```python
from build123d import *

# Parameters (mm, degrees)
SKETCH1_W           = 54
SKETCH1_H           = 32
SKETCH1_W_2         = 25
SKETCH1_H_2         = 14
BOSS_EXTRUDE1_DEPTH = 7
SKETCH2_W           = 54
SKETCH2_H           = 32
BOSS_EXTRUDE2_DEPTH = 1
CHAMFER1_SIZE       = 1


with BuildPart() as part:
    # Sketch1 → Boss-Extrude1 (new body)
    with BuildSketch(Plane(origin=(0, 0, 0), x_dir=(1, 0, 0), z_dir=(0, 1, 0))):
        with Locations((1.304347826, -0.359533527)):
            Rectangle(SKETCH1_W, SKETCH1_H)
        with Locations((-11.695652174, 7.140466473)):
            Rectangle(SKETCH1_W_2, SKETCH1_H_2, mode=Mode.SUBTRACT)
        with Locations((-11.695652174, -7.859533527)):
            Rectangle(SKETCH1_W_2, SKETCH1_H_2, mode=Mode.SUBTRACT)
        with Locations((14.304347826, 7.140466473)):
            Rectangle(SKETCH1_W_2, SKETCH1_H_2, mode=Mode.SUBTRACT)
        with Locations((14.304347826, -7.859533527)):
            Rectangle(SKETCH1_W_2, SKETCH1_H_2, mode=Mode.SUBTRACT)
    extrude(amount=BOSS_EXTRUDE1_DEPTH)

    # Sketch2 → Boss-Extrude2 (add)
    with BuildSketch(Plane.XZ):
        with Locations((1.304347826, 0.359533527)):
            Rectangle(SKETCH2_W, SKETCH2_H)
    extrude(amount=BOSS_EXTRUDE2_DEPTH)

    # Chamfer1
    chamfer1_edges = [part.edges().sort_by_distance(p)[0] for p in [
        (-25.695652174, 3, -15.640466473),
        (28.304347826, 3, -15.640466473),
        (28.304347826, 3, 16.359533527),
        (-25.695652174, 3, 16.359533527),
    ]]
    chamfer(chamfer1_edges, length=CHAMFER1_SIZE)


solid = part.part
```
Input: part model. Units: mm. Frame: model coordinates. A direction names the side the tool comes from. Give positions to 0.01 mm unless a question says otherwise; leave off trailing zeros. Loops run counter-clockwise (first coordinate to the right, second up) from the corner with the lowest first, then second, coordinate; pieces in that order, holes last.
1) Mould query, pull axis X, two halves, no side actions, for faces 3 (the flat face through (1, 7, 0)), 4 (the flat face through (-12, 0, 8)), 5 (the flat face through (27.811, 3.056, -15.133)), 6 (the flat face through (-25.189, 3.056, -15.147)). Classes: released by +X, released by -X, zero draft, split by the parting line, or undercut.
A:
face 3: zero draft
face 4: undercut
face 5: released by +X
face 6: released by -X
2) Section query C-C on y = 4.5. Return the cut outline in (x, z).
A:
outline: (-25.7, -14.64) - (-24.7, -15.64) - (27.3, -15.64) - (28.3, -14.64) - (28.3, 15.36) - (27.3, 16.36) - (-24.7, 16.36) - (-25.7, 15.36) - close; hole (-24.2, -14.14) - (0.8, -14.14) - (0.8, -0.14) - (-24.2, -0.14) - close; hole (-24.2, 0.86) - (0.8, 0.86) - (0.8, 14.86) - (-24.2, 14.86) - close; hole (1.8, -14.14) - (26.8, -14.14) - (26.8, -0.14) - (1.8, -0.14) - close; hole (1.8, 0.86) - (26.8, 0.86) - (26.8, 14.86) - (1.8, 14.86) - close
3) Section query B-B on z = 6. Return the cut outline in (x, y), and give its area (3 significant figures).
A:
outline: (-25.7, -1) - (28.3, -1) - (28.3, 7) - (26.8, 7) - (26.8, 0) - (1.8, 0) - (1.8, 7) - (0.8, 7) - (0.8, 0) - (-24.2, 0) - (-24.2, 7) - (-25.7, 7) - close
area: 82.0 mm2
4) Line query: L1, parallel to X at y = 4.75, z = -12.5; L2, parallel to Z at x = -12, y = 5; L3, parallel to Y at x = -9, z = -6.5. Output: solid intervals per line, ascending.
A:
L1: x = -25.7 to -24.2, 0.8 to 1.8, 26.8 to 28.3
L2: z = -15.64 to -14.14, -0.14 to 0.86, 14.86 to 16.36
L3: y = -1 to 0
5) Section query A-A on x = -6. Return the cut outline in (y, z).
A:
outline: (-1, -15.64) - (7, -15.64) - (7, -14.14) - (0, -14.14) - (0, -0.14) - (7, -0.14) - (7, 0.86) - (0, 0.86) - (0, 14.86) - (7, 14.86) - (7, 16.36) - (-1, 16.36) - close
6) Contact query for a flat-ended pin moving along its axis: pin 1 (4 mm diameter, centred on x = -7.5, z = -3.5, fed in from +Y). Output: stop coordinate, or through.
A:
pin 1: stops at y = 0
7) Reachability of faces 1 (the flat face through (-24.196, 3, -7)), 2 (the flat face through (1, 3, 16.36)) from +Z, -Z, +X, -X, +Y, -Y: full face, straight path, thin tool, end or side. Return the list, or none.
A:
face 1: +Y
face 2: +Z, +X, -X, +Y, -Y
